Autodesk Inventor part; units mm, degrees
ref_plane "Work Plane1" through (29, 0, 0) normal (0, -1, 0) x (1, 0, 0)
ref_plane "YZ Plane" through (0, 0, 0) normal (1, 0, 0) x (0, 1, 0)
ref_plane "XZ Plane" through (0, 0, 0) normal (0, 1, 0) x (-1, 0, 0)
sketch "Rascunho1" plane through (0, 0, 0) normal (0, 0, 1) x (1, 0, 0)
  line L0 (-2.6667, 0) -> (110, 0)
  line L1 (110, 0) -> (110, 6)
  line L2 (110, 6) -> (74, 6)
  line L3 (74, 6) -> (72.9264, 6)
  line L4 (72.9264, 6) -> (0, 6)
  line L5 (0, 6) -> (0, 9)
  line L6 (0, 9) -> (-12, 9)
  line L7 (-12, 9) -> (-12, 5.7735)
  line L8 (-12, 5.7735) -> (-6, 5.7735)
  line L9 (-6, 5.7735) -> (-2.6667, 0)
  line L10 (-34.4, 0) -> (122.4, 0)
  line L11 (0, -1.8) -> (0, 10.8)
  line L12 (74, 6) -> (0, 6) construction
  dimension "d1" = 36
  dimension "d2" = 1.0736
  dimension "d3" = 12
  dimension "d4" = 6
  dimension "d5" = 60
  dimension "d6" = 12
  dimension "d7" = 12
  dimension "d8" = 11.547
  dimension "d9" = 18
  dimension "d26" = 110
revolve "Corpo" add sketch "Rascunho1" angle 360 about axis through (-2.6667, 0, 0) along (1, 0, 0)
sketch "Rascunho2" plane through (-12, 0, 0) normal (-1, 0, 0) x (0, 0, 1)
  circle A0 centre (0, 0) radius 5.7735
  line L0 (0, -12.6) -> (0, 12.6)
  line L1 (-12.6, 0) -> (12.6, 0)
  line L2 (5.7735, 0) -> (2.8868, -5)
  line L3 (2.8868, -5) -> (-2.8868, -5)
  line L4 (-2.8868, -5) -> (-5.7735, 0)
  line L5 (-5.7735, 0) -> (-2.8868, 5)
  line L6 (-2.8868, 5) -> (2.8868, 5)
  line L7 (2.8868, 5) -> (5.7735, 0)
extrude "Fenda" add sketch "Rascunho2" against normal up to next contours L7 A0 | A0 L2 | L6 L0 A0 | A0 L0 L3 | L0 L6 A0 | A0 L3 L0 | L4 A0 | A0 L5
fillet "Raio de arredondamento1" radius 1.2 1 edges at (-12, -9, 0)
thread "Rosca"
chamfer "Chanfrar1" distance 1.0735 distance2 1.0735 1 edges at (110, -6, 0) measured on face at (110, 1.8579, 1.646)
ref_plane "Work Plane1" through (29, 0, 0) normal (0, -1, 0) x (1, 0, 0)
fillet "Fillet2" radius 0.1 1 edges at (0, -6, 0)
equation "\"d1\" = GEL"
equation "\"d3\" = KOH"
equation "\"d4\" = INTI"
equation "\"d6\" = GD"
equation "\"d7\" = BDM"
equation "\"d8\" = 1.1547 * SW"
equation "\"d9\" = KOD"
equation "\"d26\" = NLG"
equation "\"d17\" = RR"
equation "\"d13\" = GEL"
equation "\"d15\" = -0.5 * SPD + 0.5 * GD"
equation "\"d16\" = GUL"
equation "\"d30\" = R"
equation "\"GD\" = NND"
equation "\"NLG\" = 110"
equation "\"GEL\" = 36"
equation "\"KOD\" = 18"
equation "\"KOH\" = 12"
equation "\"INTI\" = 6"
equation "\"GAL\" = 0.61345 * PTC"
equation "\"GUL\" = 0.61345 * PTC"
equation "\"BDM\" = NND"
equation "\"RR\" = 1.2"
equation "\"SPD\" = NND - 1.2269 * PTC"
equation "\"R\" = 0.1"
equation "\"TOA\" = 30deg"
equation "\"GD1\" = THREADDIA - 1.2269 * PTC"
equation "\"THREADDIA\" = 12"
equation "\"FAWI\" = 45deg"
equation "\"ANG\" = 120deg"
equation "\"PTC\" = 1.75"
equation "\"NND\" = 12"
equation "\"E0\" = 1.155 * SW"
properties part number "DIN 912 - M12x110" material "Aço Inox AISI 304"
Read the model definition and answer for the solid it produces. Units are mm, in the model's axes. A direction names the side the tool comes from. Give positions to 0.01 mm unless a question says otherwise; leave off trailing zeros. Loops run counter-clockwise (first coordinate to the right, second up) from the corner with the lowest first, then second, coordinate; pieces in that order, holes last. Notation, with made-up numbers: M 65.5,-32.75 L 110.5,-32.75 A27 cw 110.5,-13.75 Z; hole C 21,27 d8. An arc over 180 degrees is marked long. Write each question's results on one line, items separated by ' | '.
1. Section A-A on x = 7.5 is taken. Give the vertices of the cut face in (y, z).
Values:
outline: C 0,0 d12
2. Straight lines are drawn through the part: line 1 (X direction, y = 4.25, z = 6); line 2 (X direction, y = 3.75, z = 1.25); line 3 (Y direction, x = 9, z = 4.75). For each, find the intervals that lie inside material, in ascending order. Write a range as [from, to].
Values:
line 1: x = [-12, 0] | line 2: x = [-4.95, 110] | line 3: y = [-3.67, 3.67]
3. A tool of negligible diameter and unlimited length cuts with its end or side. For faces 1 (the face through (54, -6, 0)), 2 (the face through (-9, -5, 0)), 3 (the face through (110, 0, 0)), from which of +Z, -Z, +X, -X, +Y, -Y can it reach the whole face along a straight path? Write none if from no direction.
Values:
face 1: +X | face 2: -X | face 3: +Z, -Z, +X, +Y, -Y
4. The mould has two halves that part along Y. Classify faces 4 (the face through (-5.476, -1.172, -8.923)), 5 (the face through (0, 2, -6)), 6 (the face through (-2.875, 0.344, -0.108)): pulls with the +Y half, pulls with the -Y half, needs draft (parallel to the pull), parting line crosses it, or undercut.
Values:
face 4: parting line crosses it | face 5: needs draft | face 6: undercut
5. Given pin 1 (2 mm diameter, centred on x = 66.5, y = -5, fed in from +Z); pin 2 (4 mm diameter, centred on x = 7.5, z = -5, fed in from +Y); pin 3 (1 mm diameter, centred on y = 0, z = 0, fed in from -X), each flat-ended and moving along its own axis, determine where each tip first touches the part or whether it passes through.
Values:
pin 1: stops at z = 4.47 | pin 2: stops at y = 5.2 | pin 3: stops at x = -2.96
